```python
from build123d import *

# Parameters (mm, degrees)
SKETCH1_R           = 11.2
BOSS_EXTRUDE1_DEPTH = 18
FILLET1_R           = 1


with BuildPart() as part:
    # Sketch1 → Boss-Extrude1 (new body)
    with BuildSketch(Plane(origin=(0, 0, 0), x_dir=(0, 0, -1), z_dir=(1, 0, 0))):
        with BuildLine():
            Line((26, 0), (30, 0))
            ThreePointArc((30, 0), (2, -28), (-26, 0))
            Line((-26, 0), (-30, 0))
            ThreePointArc((-30, 0), (-2, 28), (26, 0))
        make_face()
        Circle(SKETCH1_R, mode=Mode.SUBTRACT)
    extrude(amount=BOSS_EXTRUDE1_DEPTH)

    # Sketch2 → Revolve1 (revolve)
    with BuildSketch(Plane(origin=(0, 0, 0), x_dir=(1, 0, 0), z_dir=(0, 1, 0))):
        Polygon((0, 21.579383981), (-1, 21.579383981), (-1, 18.6), (-7.5, 18.6), (-10, 21.579383981), (-11, 21.579383981), (-11, 17.579383981), (0, 11.2), align=None)
    revolve(axis=Axis((0, 0, 0), (-1, 0, 0)))

    # Sketch4 → Revolve2 (revolve)
    with BuildSketch(Plane.XY, mode=Mode.PRIVATE) as revolve2_sk:
        Polygon((6.5, 11.2), (8.5, 9.2), (9.5, 9.2), (11.5, 11.2), align=None)
    revolve(revolve2_sk.sketch.rotate(Axis((0, 0, 0), (1, 0, 0)), 90), axis=Axis((0, 0, 0), (1, 0, 0)))

    # Fillet1
    fillet1_edges = [part.edges().sort_by_distance(p)[0] for p in [
        (0, 0, 11.2),
        (18, 0, 11.2),
        (-11, 0, 17.579383981),
        (11.5, 11.2, 0),
        (6.5, 11.2, 0),
        (8.5, 0, -9.2),
        (9.5, 0, -9.2),
    ]]
    fillet(fillet1_edges, radius=FILLET1_R)


solid = part.part
```
The model under review builds one solid part; all positions refer to its coordinate system, in mm. A direction names the side the tool comes from. Give positions to 0.01 mm unless a question says otherwise; leave off trailing zeros. Write each loop counter-clockwise with the first axis right and the second up, starting at its lowest first coordinate (ties: lowest second). Pieces come first, ordered by that corner, then holes. Notation, with made-up numbers: (2, 51) - (16, 51) arc R29 cw to (16, 86) - close; hole circle Ø8 at (-16, -32). An arc over 180 degrees is marked (long way). Answer in a Markdown table with one row per item. Add a question column.
1. Tool access review of faces 5 (the conical face through (-7.656, -5.643, -17.919)), 6 (the flat face through (9, 0, -28)), 7 (the cylindrical face through (14.42, 0.49, 11.19)), 8 (the cylindrical face through (-10.507, -6.482, -20.583)), 9 (the cylindrical face through (8.874, -27.993, -2.616)): name each direction out of +Z, -Z, +X, -X, +Y, -Y from which nothing blocks a thin tool from reaching the whole face with its end or side.
2. We need section C-C on x = -4. Write out the cut boundary in (y, z), then the cut area to 3 significant figures.
3. We need section D-D on x = -9. Write out the cut boundary in (y, z).
4. We need section B-B on y = 23. Write out the cut boundary in (x, z).
5. Draft analysis for pull direction X (two halves, no side actions). For faces 1 (the flat face through (9, 0, 28)), 2 (the flat face through (-1, -18, -6)), 3 (the flat face through (-11, 16, 10)), 4 (the flat face through (18, 13, 0)), state which applies: +X half, -X half, draft (parallel to the pull), parting line (faces both ways), or undercut.
6. We need section A-A on x = 15.5. Write out the cut boundary in (y, z).
7. Insertion check: P1, Ø21, axis at y = 0, z = 0, coming from the -X side; P2, Ø3, axis at x = -4.5, y = -5.5, coming from the -Z side; P3, Ø3, axis at x = 12.5, z = -28, coming from the +Y side. Each pin has a flat end and moves straight along its axis. Give the tip position at first contact, or say it passes through.
8. Wall thickness on line 1 along X through (y, z) = (18.5, -11.5); line 2 along Z through (x, y) = (4.25, -5.5); line 3 along Y through (x, z) = (7.5, 0.5): over which ranges is each line inside the solid? List them lowest first. Write a range as [from, to].
Ans:
| question | item | result |
|---|---|---|
| 1 | face 5 | none |
| 1 | face 6 | -Z, +X, -X, +Y |
| 1 | face 7 | +X |
| 1 | face 8 | -X |
| 1 | face 9 | +X, -X, -Y |
| 2 | outline | circle Ø37.2 at (0, 0); hole circle Ø27.04 at (0, 0) |
| 2 | area | 513 mm^2 |
| 3 | outline | circle Ø40.78 at (0, 0); hole circle Ø32.84 at (0, 0) |
| 4 | outline | (0, -13.97) - (18, -13.97) - (18, 17.97) - (0, 17.97) - close |
| 5 | face 1 | draft |
| 5 | face 2 | undercut |
| 5 | face 3 | -X half |
| 5 | face 4 | +X half |
| 6 | outline | (0, -30) - (0, -26) arc R28 ccw to (0, 30) - (0, 26) arc R28 ccw to start; hole circle Ø22.4 at (0, 0) |
| 7 | P1 | stops at x = 7.2 |
| 7 | P2 | stops at z = -18.16 |
| 7 | P3 | stops at y = 0 |
| 8 | line 1 | x = [0, 18] |
| 8 | line 2 | z = [-29.45, -9.76], [9.76, 25.45] |
| 8 | line 3 | y = [-27.89, -10.19], [10.19, 27.96] |
